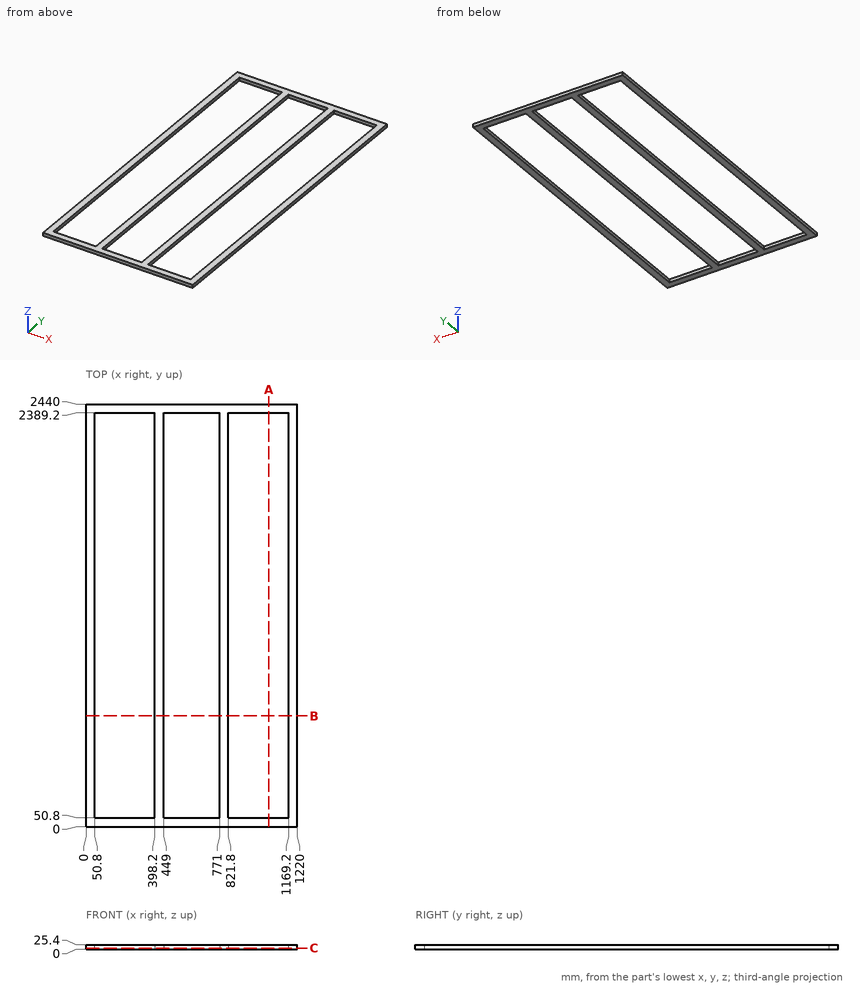
Part print with two shaded views. Sizes in mm from the minimum x, y, z corner. Round coordinates to 2 decimals unless told otherwise and drop trailing zeros. Order: outer loops, then holes, each group sorted by start corner. A loop starts at its lowest first (then second) coordinate and runs counter-clockwise, first axis right, second up. Notation, with made-up numbers: M 12,-39.75 L 23,-39.75 A26 ccw 23,-17.75 Z; hole C 42.25,66.5 d9. An arc over 180 degrees is marked long. Answer in a Markdown table with one row per item. Add a question column.
Q1. Cut at C-C on z = 5.5. Give the cut face in (x, y).
Q2. Cut at A-A on x = 1055. Give the cut face in (y, z).
Q3. Wall check: L1, parallel to X at y = 286, z = 20.25; L2, parallel to Y at x = 625.5, z = 19.5. Give the ranges that are in metal, low to high. Write a range as from..to.
Q4. Cut at B-B on y = 639. Give the cut face in (x, z).
Q5. Pin check, flat tip, straight feed: pin 1 (1 mm diameter, centred on x = 526, z = 20.5, fed in from -Y). Stop position of the tip, or through.
Established:
| question | item | result |
|---|---|---|
| 1 | outline | M 0,0 L 1220,0 L 1220,2440 L 0,2440 Z; hole M 50.8,50.8 L 398.2,50.8 L 398.2,2389.2 L 50.8,2389.2 Z; hole M 449,50.8 L 771,50.8 L 771,2389.2 L 449,2389.2 Z; hole M 821.8,50.8 L 1169.2,50.8 L 1169.2,2389.2 L 821.8,2389.2 Z |
| 2 | outline | M 0,0 L 50.8,0 L 50.8,25.4 L 0,25.4 Z; M 2389.2,0 L 2440,0 L 2440,25.4 L 2389.2,25.4 Z |
| 3 | L1 | x = 0..50.8, 398.2..449, 771..821.8, 1169.2..1220 |
| 3 | L2 | y = 0..50.8, 2389.2..2440 |
| 4 | outline | M 0,0 L 50.8,0 L 50.8,25.4 L 0,25.4 Z; M 398.2,0 L 449,0 L 449,25.4 L 398.2,25.4 Z; M 771,0 L 821.8,0 L 821.8,25.4 L 771,25.4 Z; M 1169.2,0 L 1220,0 L 1220,25.4 L 1169.2,25.4 Z |
| 5 | pin 1 | stops at y = 0 |
